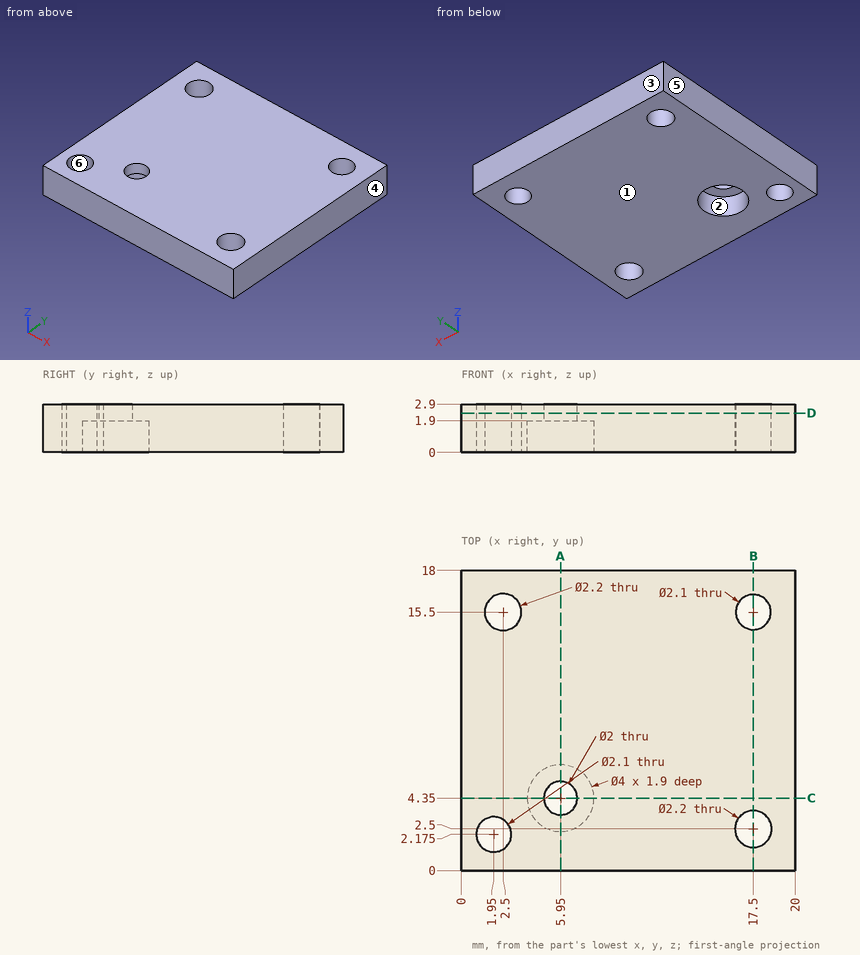
Part print with two shaded views. Sizes in mm from the minimum x, y, z corner. A direction names the side the tool comes from. Round coordinates to 2 decimals unless told otherwise and drop trailing zeros. Loops run counter-clockwise (first coordinate to the right, second up) from the corner with the lowest first, then second, coordinate; pieces in that order, holes last.
Item 1: Saw through at D-D (z = 2.35). List the corners of the cut face in (x, y) (3 decimals).
Item 2: Two-plate mould, pull along X, no slides. Class the marked faces 3, 4, 5 and 6: released by +X, released by -X, zero draft, split by the parting line, or undercut.
Item 3: Saw through at B-B (x = 17.5). List the corners of the cut face in (y, z), then the cut area to 3 significant figures.
Item 4: Pin check, flat tip, straight feed: P1, Ø1.7, axis at x = 1.95, y = 2.175, coming from the -Z side. Stop position of the tip, or through.
Item 5: Saw through at A-A (x = 5.95). List the corners of the cut face in (y, z), then the cut area to 3 significant figures.
Item 6: Saw through at C-C (y = 4.35). List the corners of the cut face in (x, z), then the cut area to 3 significant figures.
Item 7: Drill centre lines: line 1 along Y through (x, z) = (17.5, 2.2); line 2 along X through (y, z) = (1.75, 1.75); line 3 along X through (y, z) = (5, 1.25). Where is each one in solid material? Low to high.
Item 8: Which spindle directions (+Z, -Z, +X, -X, +Y, -Y) get a long thin tool onto all of the face, cutting with end or side? Do the marked faces 1 and 2. Say none if no direction does.
Worked answers:
1. outline: (0, 0) - (20, 0) - (20, 18) - (0, 18) - close; hole circle Ø2.1 at (1.95, 2.175); hole circle Ø2.2 at (2.5, 15.5); hole circle Ø2 at (5.95, 4.35); hole circle Ø2.2 at (17.5, 2.5); hole circle Ø2.1 at (17.5, 15.5)
2. face 3: zero draft
2. face 4: released by +X
2. face 5: released by -X
2. face 6: undercut
3. outline: (0, 0) - (1.4, 0) - (1.4, 2.9) - (0, 2.9) - close; (3.6, 0) - (14.45, 0) - (14.45, 2.9) - (3.6, 2.9) - close; (16.55, 0) - (18, 0) - (18, 2.9) - (16.55, 2.9) - close
3. area: 39.7 mm2
4. P1: passes through
5. outline: (0, 0) - (2.35, 0) - (2.35, 1.9) - (3.35, 1.9) - (3.35, 2.9) - (0, 2.9) - close; (5.35, 1.9) - (6.35, 1.9) - (6.35, 0) - (18, 0) - (18, 2.9) - (5.35, 2.9) - close
5. area: 42.6 mm2
6. outline: (0, 0) - (3.95, 0) - (3.95, 1.9) - (4.95, 1.9) - (4.95, 2.9) - (0, 2.9) - close; (6.95, 1.9) - (7.95, 1.9) - (7.95, 0) - (20, 0) - (20, 2.9) - (6.95, 2.9) - close
6. area: 48.4 mm2
7. line 1: y = 0 to 1.4, 3.6 to 14.45, 16.55 to 18
7. line 2: x = 0 to 0.99, 2.91 to 16.7, 18.3 to 20
7. line 3: x = 0 to 4.06, 7.84 to 20
8. face 1: -Z, +X, -X, +Y, -Y
8. face 2: -Z
